```python
from build123d import *

# Parameters (mm, degrees)
BOSS_EXTRUDE1_DEPTH = 31.75
CUT_EXTRUDE2_START  = -3.175
CUT_EXTRUDE2_DEPTH  = 25.4
SKETCH4_W           = 25.4
SKETCH4_H           = 25.4
CUT_EXTRUDE3_DEPTH  = 3.175
SKETCH6_W           = 25.4
SKETCH6_H           = 25.4
CUT_EXTRUDE5_DEPTH  = 3.175
FILLET1_R           = 5
CUT_EXTRUDE6_REACH  = 79.895
SKETCH8_R           = 3.175
CUT_EXTRUDE7_REACH  = 69.69
SKETCH9_R           = 3.175


with BuildPart() as part:
    # Sketch1 → Boss-Extrude1 (new body)
    with BuildSketch(Plane(origin=(0, 0, 0), x_dir=(0, 0, -1), z_dir=(1, 0, 0))):
        with BuildLine():
            Line((15.875, 42.5), (-15.875, 42.5))
            Line((-15.875, 42.5), (-15.875, 0))
            Line((-15.875, 0), (-38.855970389, -22.980970389))
            Line((-38.855970389, -22.980970389), (-16.405330086, -45.431610691))
            Line((-16.405330086, -45.431610691), (6.575640303, -22.450640303))
            ThreePointArc((6.575640303, -22.450640303), (13.458175157, -12.150198978), (15.875, 0))
            Line((15.875, 0), (15.875, 42.5))
        make_face()
    extrude(amount=BOSS_EXTRUDE1_DEPTH)

    # Sketch3 → Cut-Extrude2 (cut)
    with BuildSketch(Plane.ZY.offset(CUT_EXTRUDE2_START)):
        with BuildLine():
            Line((16.405330086, -40.941482631), (34.365842328, -22.980970389))
            Line((34.365842328, -22.980970389), (12.7, -1.315128061))
            Line((12.7, -1.315128061), (12.7, 39.325))
            Line((12.7, 39.325), (-12.7, 39.325))
            Line((-12.7, 39.325), (-12.7, 0))
            ThreePointArc((-12.7, 0), (-10.524857642, -10.93517908), (-4.330576272, -20.205576272))
            Line((-4.330576272, -20.205576272), (16.405330086, -40.941482631))
        make_face()
    extrude(amount=-CUT_EXTRUDE2_DEPTH, mode=Mode.SUBTRACT)

    # Sketch4 → Cut-Extrude3 (cut)
    with BuildSketch(Plane(origin=(0, 42.5, 0), x_dir=(1, 0, 0), z_dir=(0, 1, 0))):
        with Locations((15.875, 0)):
            Rectangle(SKETCH4_W, SKETCH4_H)
    extrude(amount=-CUT_EXTRUDE3_DEPTH, mode=Mode.SUBTRACT)

    # Sketch6 → Cut-Extrude5 (cut)
    with BuildSketch(Plane(origin=(0, -30.918470389, 30.918470389), x_dir=(1, 0, 0), z_dir=(0, -0.7071067811865518, 0.7071067811865434))):
        with Locations((15.875, -4.649679849)):
            Rectangle(SKETCH6_W, SKETCH6_H)
    extrude(amount=-CUT_EXTRUDE5_DEPTH, mode=Mode.SUBTRACT)

    # Fillet1
    fillet1_edges = [part.edges().sort_by_distance(p)[0] for p in [
        (15.875, 0, 15.875),
        (15.875, -1.315128061, 12.7),
    ]]
    fillet(fillet1_edges, radius=FILLET1_R)

    # Cut-Extrude6: up to this face of the body (flat: up to its plane)
    cut_extrude6_end = Plane(part.part.faces().sort_by_distance((15.875, 22.285533906, 15.875))[0])
    # Sketch8 → Cut-Extrude6 (cut, up to the picked face)
    with BuildSketch(Plane(origin=(0, 0, -15.875), x_dir=(-1, 0, 0), z_dir=(0, 0, -1)), mode=Mode.PRIVATE) as cut_extrude6_sk1:
        with Locations((-15.875, 23.45)):
            Circle(SKETCH8_R)
    cut_extrude6_tool1 = split(extrude(cut_extrude6_sk1.sketch, amount=-CUT_EXTRUDE6_REACH, mode=Mode.PRIVATE), bisect_by=cut_extrude6_end, keep=Keep.BOTH, mode=Mode.PRIVATE)
    add(cut_extrude6_tool1.solids().sort_by(Axis((15.875, 23.45, -15.875), (0, 0, 1)))[0], mode=Mode.SUBTRACT)

    # Cut-Extrude7: up to this face of the body (flat: up to its plane)
    cut_extrude7_end = Plane(part.part.faces().sort_by_distance((0, 0.759502888, 5.54562078))[0])
    # Sketch9 → Cut-Extrude7 (cut, up to the picked face)
    with BuildSketch(Plane(origin=(31.75, 0, 0), x_dir=(0, 0, -1), z_dir=(1, 0, 0)), mode=Mode.PRIVATE) as cut_extrude7_sk1:
        with Locations(Location((-14.160266056, -20.735906358, 0), (0, 0, 180))):
            Circle(SKETCH9_R)
    cut_extrude7_tool1 = split(extrude(cut_extrude7_sk1.sketch, amount=-CUT_EXTRUDE7_REACH, mode=Mode.PRIVATE), bisect_by=cut_extrude7_end, keep=Keep.BOTH, mode=Mode.PRIVATE)
    add(cut_extrude7_tool1.solids().sort_by(Axis((31.75, -20.735906, 14.160266), (-1, 0, 0)))[0], mode=Mode.SUBTRACT)


solid = part.part
```
Build history of the part. All positions in model axes, mm. A direction names the side the tool comes from. Round coordinates to 2 decimals unless told otherwise and drop trailing zeros. Write each loop counter-clockwise with the first axis right and the second up, starting at its lowest first coordinate (ties: lowest second). Pieces come first, ordered by that corner, then holes. Notation, with made-up numbers: (66, 32.5) -> (123, 32.5) arc R15 cw to (123, 40.5) -> close; hole circle Ø8 at (-4, 79). An arc over 180 degrees is marked (long way). Put each result on its own line as item: value.
Item 1: Slice it at D-D, the plane x = 15. Give the cut face in (y, z) (3 decimals).
Here are the results:
outline: (-45.432, 16.405) -> (-22.451, -6.576) arc R31.75 ccw to (0, -15.875) -> (20.398, -15.875) -> (20.398, -12.7) -> (0, -12.7) arc R28.575 cw to (-20.206, -4.331) -> (-43.187, 18.65) -> close; (-25.226, 36.611) -> (-2.78, 14.164) arc R5 ccw to (0.756, 12.7) -> (20.398, 12.7) -> (20.398, 15.875) -> (2.071, 15.875) arc R5 cw to (-1.464, 17.339) -> (-22.981, 38.856) -> close; (26.502, -15.875) -> (42.5, -15.875) -> (42.5, -12.7) -> (26.502, -12.7) -> close; (26.502, 12.7) -> (42.5, 12.7) -> (42.5, 15.875) -> (26.502, 15.875) -> close
Item 2: Tool access for faces 1 (the face through (12.9, 21.5, -12.7)), 2 (the face through (1.61, -17.636, 13.472)), 3 (the face through (12, 23, 15.875)), 4 (the face through (28.575, 0, 7)), 5 (the face through (31.75, -1, 6)): list every direction of +Z, -Z, +X, -X, +Y, -Y with a clear straight run to the whole face (end or side of a thin tool).
Here are the results:
face 1: +Y
face 2: +X, -X
face 3: +Z, +X, -X, +Y
face 4: none
face 5: +Z, -Z, +X, +Y, -Y
Item 3: Flat gauge pins, fed straight in: P1, Ø8, axis at y = -23.5, z = 26.5, coming from the -X side; P2, Ø12, axis at x = 9.5, z = 23.5, coming from the -Y side; P3, Ø5, axis at x = 19.5, z = 11, coming from the -Y side; P4, Ø5, axis at x = 23.5, y = 0, coming from the +Z side (3 decimals). Where does each tip first touch, or does it go through?
Here are the results:
P1: stops at x = 0
P2: stops at y = -44.34
P3: stops at y = -42.53
P4: stops at z = 18.375
Item 4: Slice it at A-A, the plane y = 23.45. Give the cut face in (x, z) (3 decimals), plus the area to 3 significant figures.
Here are the results:
outline: (0, -15.875) -> (12.7, -15.875) -> (12.7, -12.7) -> (3.175, -12.7) -> (3.175, 12.7) -> (12.7, 12.7) -> (12.7, 15.875) -> (0, 15.875) -> close; (19.05, -15.875) -> (31.75, -15.875) -> (31.75, 15.875) -> (19.05, 15.875) -> (19.05, 12.7) -> (28.575, 12.7) -> (28.575, -12.7) -> (19.05, -12.7) -> close
area: 323 mm^2
Item 5: Slice it at C-C, the plane y = 5. Give the cut face in (x, z) (3 decimals).
Here are the results:
outline: (0, -15.875) -> (31.75, -15.875) -> (31.75, 15.875) -> (0, 15.875) -> close; hole (3.175, -12.7) -> (28.575, -12.7) -> (28.575, 12.7) -> (3.175, 12.7) -> close
Item 6: Wall check: probe 1 along Z at (x, y) = (13, 38) (3 decimals); probe 2 along X at (y, z) = (6.5, 8) (3 decimals); probe 3 along Z at (x, y) = (29, 12.5) (3 decimals). Give the ranges that are in metal, low to high. Write a range as from..to.
Here are the results:
probe 1: z = -15.875..-12.7, 12.7..15.875
probe 2: x = 0..3.175, 28.575..31.75
probe 3: z = -15.875..15.875
Item 7: Two-plate mould, pull along Y, no slides. Class faces 6 (the face through (16.05, -1.13, 13.07)), 7 (the face through (15.65, -12.31, -13.39)), 8 (the face through (12.847, 24.404, 14.265)), 9 (the face through (16, 42.5, -14)): pulls with the +Y half, pulls with the -Y half, needs draft (parallel to the pull), parting line crosses it, or undercut.
Here are the results:
face 6: undercut
face 7: pulls with the -Y half
face 8: undercut
face 9: pulls with the +Y half
Item 8: Slice it at B-B, the plane x = 6.5. Give the cut face in (y, z) (3 decimals), plus the area to 3 significant figures.
Here are the results:
outline: (-45.432, 16.405) -> (-22.451, -6.576) arc R31.75 ccw to (0, -15.875) -> (42.5, -15.875) -> (42.5, -12.7) -> (0, -12.7) arc R28.575 cw to (-20.206, -4.331) -> (-43.187, 18.65) -> close; (-25.226, 36.611) -> (-2.78, 14.164) arc R5 ccw to (0.756, 12.7) -> (42.5, 12.7) -> (42.5, 15.875) -> (2.071, 15.875) arc R5 cw to (-1.464, 17.339) -> (-22.981, 38.856) -> close
area: 556 mm^2
